Print and shaded views of the part. All mm, measured from the part's lowest x, y and z. A direction names the side the tool comes from. Coordinates: 2 decimals unless noted, no trailing zeros. Loops run counter-clockwise (first coordinate to the right, second up) from the corner with the lowest first, then second, coordinate; pieces in that order, holes last. Notation, with made-up numbers: (60, 65) -> (83, 65) arc R8 cw to (83, 78) -> close; hole circle Ø6 at (6.5, 5.5). An arc over 180 degrees is marked (long way). One line per question, with ' | ' between items. Start each with the question number.
1) Cut at A-A (x = 11.25). List the corners of the cut face in (y, z).
2) Cut at B-B (z = 3.75). List the corners of the cut face in (x, y).
3) Two-plate mould, pull along Z, no slides. Class the marked faces 1, 2 and 3: released by +Z, released by -Z, zero draft, split by the parting line, or undercut.
4) Probe L1, parallel to X at y = 3.8, z = 11.25; L2, parallel to X at y = 3.95, z = 5. List the from-to ranges inside material, lowest first. Write a range as from..to.
5) Cut at C-C (y = 3.25). Count the separate pieces of the cut face and the enclosed holes in it, plus the area to 3 significant figures.
6) 3-axis set-ups, long thin cutter, end or side, ignore diameter. For the marked faces 4 and 5: which of +Z, -Z, +X, -X, +Y, -Y reach the whole face in a straight line?
7) Cut at D-D (x = 3.75). List the corners of the cut face in (y, z).
8) Drop a flat-ended pin along its axis: pin 1 (2.5 mm diameter, centred on x = 11.25, z = 11.25, fed in from +Y). Give the stop position or say it passes through.
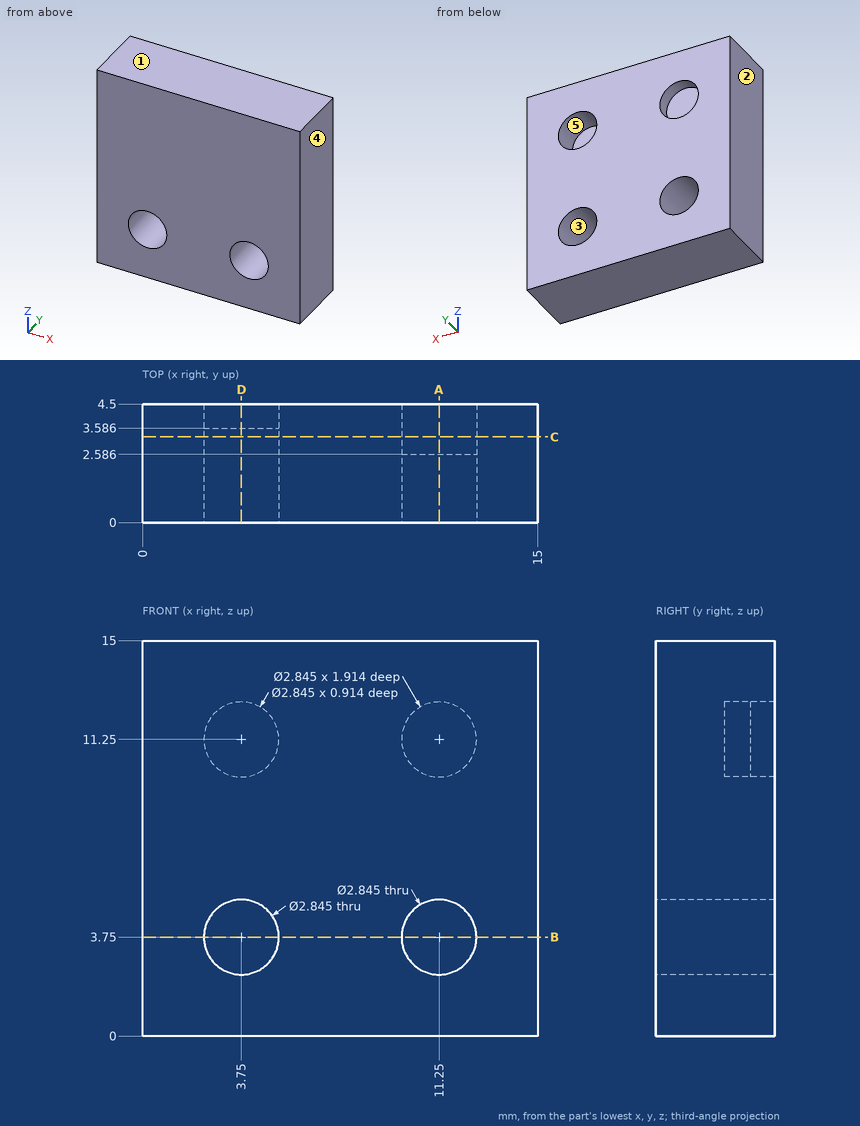
Reported:
1) outline: (0, 0) -> (4.5, 0) -> (4.5, 2.33) -> (0, 2.33) -> close; (0, 5.17) -> (4.5, 5.17) -> (4.5, 9.83) -> (2.59, 9.83) -> (2.59, 12.67) -> (4.5, 12.67) -> (4.5, 15) -> (0, 15) -> close
2) outline: (0, 0) -> (2.33, 0) -> (2.33, 4.5) -> (0, 4.5) -> close; (5.17, 0) -> (9.83, 0) -> (9.83, 4.5) -> (5.17, 4.5) -> close; (12.67, 0) -> (15, 0) -> (15, 4.5) -> (12.67, 4.5) -> close
3) face 1: released by +Z | face 2: zero draft | face 3: undercut
4) L1: x = 0..2.33, 5.17..9.83, 12.67..15 | L2: x = 0..3.07, 4.43..10.57, 11.93..15
5) separate pieces: 1 | enclosed holes: 3 | area: 206 mm²
6) face 4: +Z, -Z, +X, +Y, -Y | face 5: +Y
7) outline: (0, 0) -> (4.5, 0) -> (4.5, 2.33) -> (0, 2.33) -> close; (0, 5.17) -> (4.5, 5.17) -> (4.5, 9.83) -> (3.59, 9.83) -> (3.59, 12.67) -> (4.5, 12.67) -> (4.5, 15) -> (0, 15) -> close
8) pin 1: stops at y = 2.59
